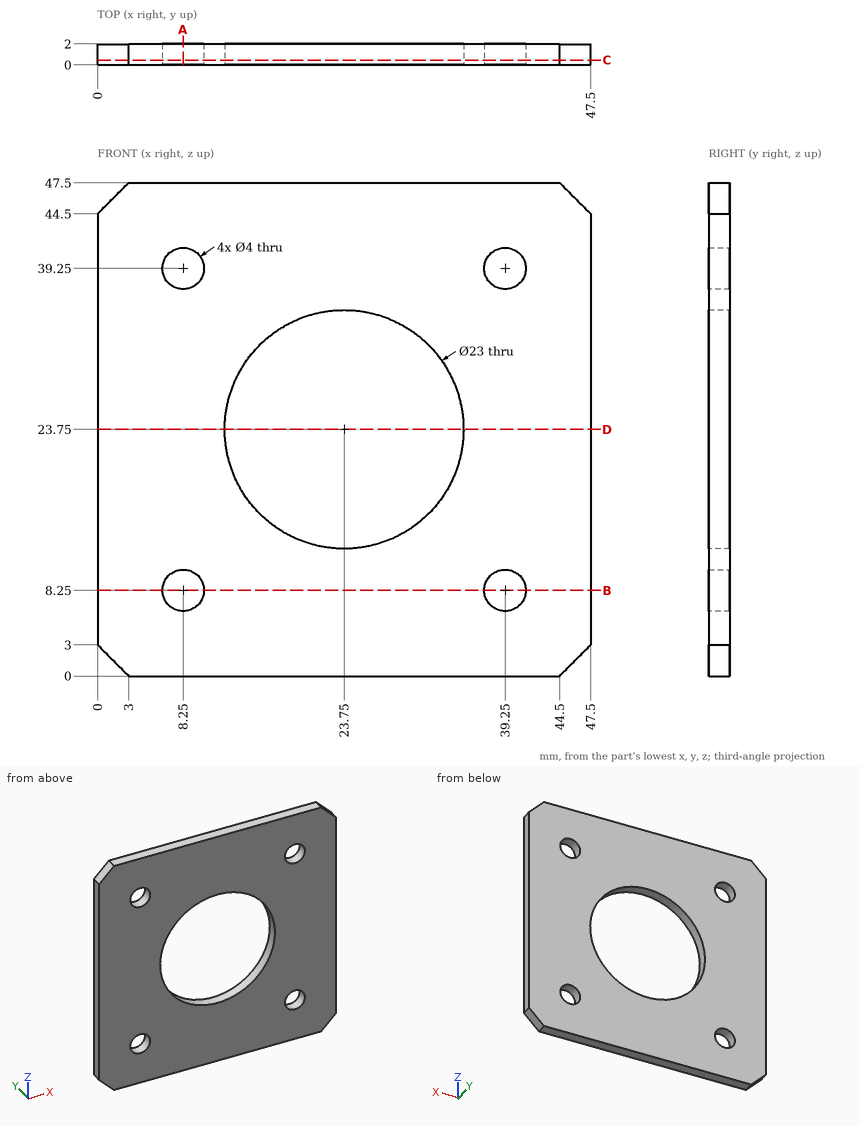
Print and shaded views of the part. All mm, measured from the part's lowest x, y and z. Give positions to 0.01 mm unless a question says otherwise; leave off trailing zeros. Loops run counter-clockwise (first coordinate to the right, second up) from the corner with the lowest first, then second, coordinate; pieces in that order, holes last. Notation, with made-up numbers: (42, 88.25) -> (81, 88.25) arc R20 ccw to (81, 98.25) -> close; hole circle Ø11 at (79.5, 21.25). An arc over 180 degrees is marked (long way). Use a Markdown table: item, result.
1. Slice it at A-A (x = 8.25). List the corners of the cut face in (y, z), plus the area to 3 significant figures.
Check result:
| item | result |
|---|---|
| outline | (0, 0) -> (2, 0) -> (2, 6.25) -> (0, 6.25) -> close; (0, 10.25) -> (2, 10.25) -> (2, 37.25) -> (0, 37.25) -> close; (0, 41.25) -> (2, 41.25) -> (2, 47.5) -> (0, 47.5) -> close |
| area | 79.0 mm^2 |
2. Slice it at C-C (y = 0.45). List the corners of the cut face in (x, z), plus the area to 3 significant figures.
Check result:
| item | result |
|---|---|
| outline | (0, 3) -> (3, 0) -> (44.5, 0) -> (47.5, 3) -> (47.5, 44.5) -> (44.5, 47.5) -> (3, 47.5) -> (0, 44.5) -> close; hole circle Ø4 at (8.25, 8.25); hole circle Ø4 at (8.25, 39.25); hole circle Ø23 at (23.75, 23.75); hole circle Ø4 at (39.25, 8.25); hole circle Ø4 at (39.25, 39.25) |
| area | 1,770 mm^2 |
3. Wall check: L1, parallel to X at y = 0.6, z = 8.25; L2, parallel to X at y = 1.9, z = 7.5; L3, parallel to X at y = 0.45, z = 23.75. Give the ranges that are in metal, low to high. Write a range as [from, to].
Check result:
| item | result |
|---|---|
| L1 | x = [0, 6.25], [10.25, 37.25], [41.25, 47.5] |
| L2 | x = [0, 6.4], [10.1, 37.4], [41.1, 47.5] |
| L3 | x = [0, 12.25], [35.25, 47.5] |
4. Slice it at D-D (z = 23.75). List the corners of the cut face in (x, y).
Check result:
| item | result |
|---|---|
| outline | (0, 0) -> (12.25, 0) -> (12.25, 2) -> (0, 2) -> close; (35.25, 0) -> (47.5, 0) -> (47.5, 2) -> (35.25, 2) -> close |
5. Slice it at B-B (z = 8.25). List the corners of the cut face in (x, y).
Check result:
| item | result |
|---|---|
| outline | (0, 0) -> (6.25, 0) -> (6.25, 2) -> (0, 2) -> close; (10.25, 0) -> (37.25, 0) -> (37.25, 2) -> (10.25, 2) -> close; (41.25, 0) -> (47.5, 0) -> (47.5, 2) -> (41.25, 2) -> close |
